Source: three-view drawing plus pictorial views. Frame: mm from the lowest corner of the part. Round coordinates to 2 decimals unless told otherwise and drop trailing zeros. Loops run counter-clockwise (first coordinate to the right, second up) from the corner with the lowest first, then second, coordinate; pieces in that order, holes last. Notation, with made-up numbers: (29, 46.25) -> (47, 46.25) arc R9 ccw to (47, 62.25) -> close; hole circle Ø10 at (-5.75, 47). An arc over 180 degrees is marked (long way). Answer as a JSON object with one key per item and string values. Group by question number.
Item 1: Section query C-C on y = 46.5. Return loops of the section in (x, z), and give its area (3 significant figures).
Item 2: Section query A-A on x = 43. Return loops of the section in (y, z).
Item 3: Section query D-D on z = 38. Return loops of the section in (x, y).
Item 4: Section query B-B on z = 32.5. Return loops of the section in (x, y), and give its area (3 significant figures).
Item 5: Material intervals for line 1 (Z direction, x = 43, y = 7); line 2 (Y direction, x = 71, z = 47) (1 decimal); line 3 (Y direction, x = 43, z = 47), sorted ascending. Write a range as [from, to].
Item 6: Pin query (flat end, axial travel): pin 1 (10 mm diameter, centred on y = 34, z = 19, fed in from -X) (1 decimal); pin 2 (10 mm diameter, centred on x = 22, z = 15, fed in from +Y); pin 3 (5 mm diameter, centred on x = 67.5, z = 21, fed in from -Y) (1 decimal). Return the tip coordinate at first contact, or that it passes through.
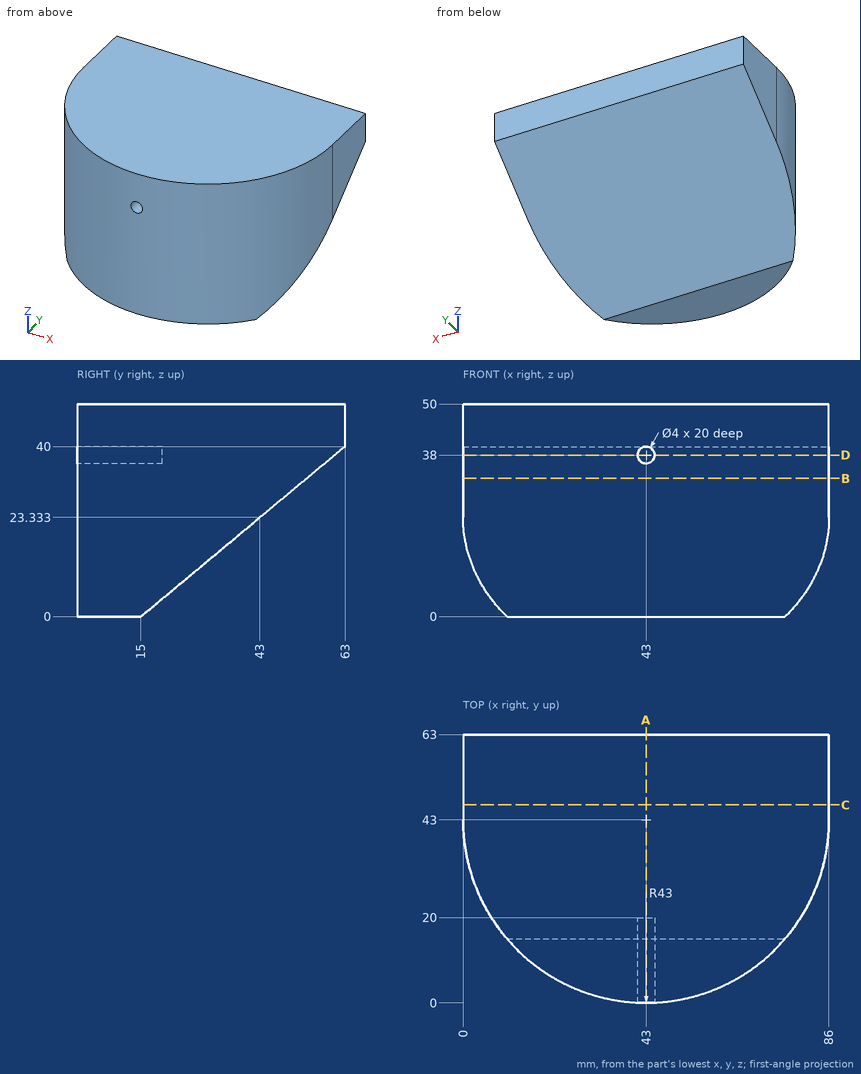
Solved:
{
 "1": {"outline": "(0, 26.25) -> (86, 26.25) -> (86, 50) -> (0, 50) -> close", "area": "2,040 mm²"},
 "2": {"outline": "(0, 0) -> (15, 0) -> (63, 40) -> (63, 50) -> (0, 50) -> (0, 40) -> (20, 40) -> (20, 36) -> (0, 36) -> close"},
 "3": {"outline": "(0, 43) arc R43 ccw to (41, 0.05) -> (41, 20) -> (45, 20) -> (45, 0.05) arc R43 ccw to (86, 43) -> (86, 60.6) -> (0, 60.6) -> close"},
 "4": {"outline": "(0, 43) arc R43 ccw to (86, 43) -> (86, 54) -> (0, 54) -> close", "area": "3,850 mm²"},
 "5": {"line 1": "[0, 36], [40, 50]", "line 2": "[10.4, 63]", "line 3": "[0, 63]"},
 "6": {"pin 1": "x = 0.2", "pin 2": "y = 39", "pin 3": "y = 6.1"}
}
